The figure shows three views and two pictorial views of one solid part (mm, origin at its lowest corner). Answer the questions. Give positions to 0.01 mm unless a question says otherwise; leave off trailing zeros. Order: outer loops, then holes, each group sorted by start corner. A loop starts at its lowest first (then second) coordinate and runs counter-clockwise, first axis right, second up. Notation, with made-up numbers: M 84,77 L 99,77 A22 cw 99,102 Z; hole C 9,1.5 d9. An arc over 180 degrees is marked long. Answer as a JSON object with one key per item and string values. Group by question number.
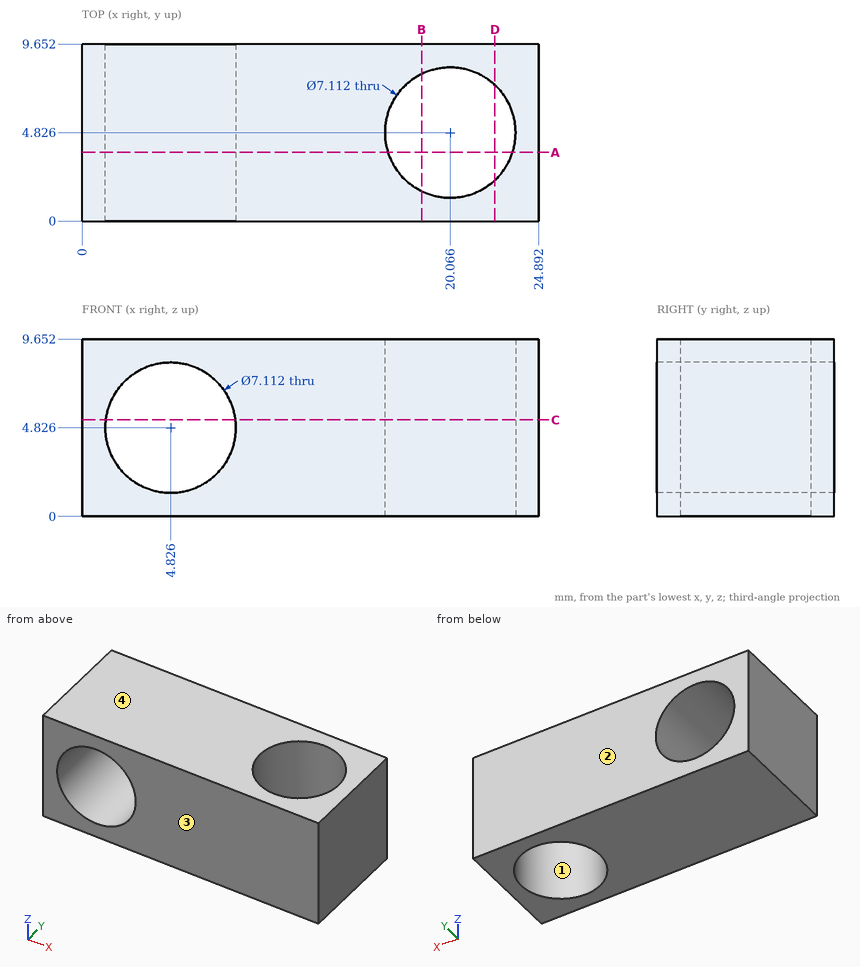
Item 1: Consider probe 1 along Z at (x, y) = (4.75, 2); probe 2 along X at (y, z) = (6.5, 5); probe 3 along X at (y, z) = (2, 6). Determine where each line is inside the solid, lowest interval first. Write a range as from..to.
Item 2: Section D-D (x = 22.5) is taken. Determine the outline of the cut face in (y, z).
Item 3: Section C-C (z = 5.25) is taken. Determine the outline of the cut face in (x, y).
Item 4: Section B-B (x = 18.5) is taken. Determine the outline of the cut face in (y, z).
Item 5: Section A-A (y = 3.75) is taken. Determine the outline of the cut face in (x, z).
Item 6: Determine the mould class of the marked faces 1, 2, 3 and 4 for opening direction Y: released by +Y, released by -Y, zero draft, split by the parting line, or undercut.
Values found:
{
 "1": {"probe 1": "z = 0..1.27, 8.38..9.65", "probe 2": "x = 0..1.27, 8.38..16.93, 23.2..24.89", "probe 3": "x = 0..1.47, 8.18..17.91, 22.22..24.89"},
 "2": {"outline": "M 0,0 L 2.23,0 L 2.23,9.65 L 0,9.65 Z; M 7.42,0 L 9.65,0 L 9.65,9.65 L 7.42,9.65 Z"},
 "3": {"outline": "M 0,0 L 1.3,0 L 1.3,9.65 L 0,9.65 Z; M 8.36,0 L 24.89,0 L 24.89,9.65 L 8.36,9.65 Z; hole C 20.07,4.83 d7.11"},
 "4": {"outline": "M 0,0 L 1.63,0 L 1.63,9.65 L 0,9.65 Z; M 8.02,0 L 9.65,0 L 9.65,9.65 L 8.02,9.65 Z"},
 "5": {"outline": "M 0,0 L 16.68,0 L 16.68,9.65 L 0,9.65 Z; M 23.46,0 L 24.89,0 L 24.89,9.65 L 23.46,9.65 Z; hole C 4.83,4.83 d7.11"},
 "6": {"face 1": "undercut", "face 2": "released by +Y", "face 3": "released by -Y", "face 4": "zero draft"}
}
